```python
from build123d import *

# Parameters (mm, degrees)
F0_R     = 17.4093828925
F1_DEPTH = 25.4
F2_W     = 27.6633873582
F2_H     = 53.7356156856
F3_DEPTH = 25.4
F4_W     = 27.6633873582
F4_H     = 17.2435138375
F5_DEPTH = 12.7


with BuildPart() as f1:
    # F0 (on Top) → F1 (new body)
    with BuildSketch(Plane.XY):
        with BuildLine():
            ThreePointArc((-62.1633082628, 0), (-54.3854373577, -19.1652168316), (-35.2955013514, -27.1260682493))
            Line((-35.2955013514, -27.1260682493), (41.6988097131, -27.1260682493))
            Line((41.6988097131, -27.1260682493), (41.6988097131, 26.6095474362))
            Line((41.6988097131, 26.6095474362), (-35.6965139508, 26.6095474362))
            ThreePointArc((-35.6965139508, 26.6095474362), (-54.3456505922, 18.6914592057), (-62.1633082628, 0))
        make_face()
        with Locations((-35.2949523061, -0.2570371656)):
            Circle(F0_R, mode=Mode.SUBTRACT)
    extrude(amount=F1_DEPTH)

    # F2 (on face) → F3 (join)
    with BuildSketch(Plane(origin=(0, 0, 0), x_dir=(1, 0, 0), z_dir=(0, 0, -1))):
        with Locations((27.867116034, 0.2582604066)):
            Rectangle(F2_W, F2_H)
    extrude(amount=F3_DEPTH)

    # F4 (on face) → F5 (cut)
    with BuildSketch(Plane(origin=(0, 0, -25.4), x_dir=(1, 0, 0), z_dir=(0, 0, -1))):
        with Locations((27.867116034, 18.5043113306)):
            Rectangle(F4_W, F4_H)
    extrude(amount=-F5_DEPTH, mode=Mode.SUBTRACT)


solid = f1.part
```
For this review, take the finished solid that the model builds, in its own axes (mm). A direction names the side the tool comes from. Coordinates: 2 decimals unless noted, no trailing zeros. Write each loop counter-clockwise with the first axis right and the second up, starting at its lowest first coordinate (ties: lowest second). Pieces come first, ordered by that corner, then holes. Notation, with made-up numbers: (6.5, 2.25) -> (19.5, 2.25) arc R27 cw to (19.5, 25.25) -> close; hole circle Ø11 at (38, 15). An arc over 180 degrees is marked (long way). Put each result on its own line as item: value.
Q1. Take a section at C-C, the plane z = 4. State the section outline as (x, y) points.
From the geometry:
outline: (-62.16, 0) arc R26.87 ccw to (-35.3, -27.13) -> (41.7, -27.13) -> (41.7, 26.61) -> (-35.7, 26.61) arc R26.87 ccw to start; hole circle Ø34.82 at (-35.29, -0.26)
Q2. Clearance check with flat-ended pins moving along their axes: pin 1 Ø10 at (x, z) = (12, -13) entering from -Y; pin 2 Ø1.5 at (x, y) = (12, 11) entering from -Z; pin 3 Ø12.5 at (y, z) = (-2, -11) entering from -X; pin 4 Ø1.5 at (y, z) = (2.5, 8) entering from -X. State where each tip first meets the part, or that it passes through.
From the geometry:
pin 1: stops at y = -27.13
pin 2: stops at z = 0
pin 3: stops at x = 14.04
pin 4: stops at x = -62.09
Q3. Tool access review of faces 5 (the flat face through (28, 8, -25.4)), 6 (the flat face through (28, -9.883, -19)), 7 (the flat face through (-16, 0, 0)): name each direction out of +Z, -Z, +X, -X, +Y, -Y from which nothing blocks a thin tool from reaching the whole face with its end or side.
From the geometry:
face 5: -Z, +X, -X, +Y, -Y
face 6: -Z, +X, -X, -Y
face 7: -Z, -X, +Y, -Y
Q4. Take a section at D-D, the plane y = 15.5. State the section outline as (x, z) points.
From the geometry:
outline: (-57.06, 0) -> (-42.7, 0) -> (-42.7, 25.4) -> (-57.06, 25.4) -> close; (-27.89, 0) -> (14.04, 0) -> (14.04, -25.4) -> (41.7, -25.4) -> (41.7, 25.4) -> (-27.89, 25.4) -> close
Q5. Take a section at A-A, the plane y = -14. State the section outline as (x, z) points, then the cut area to 3 significant figures.
From the geometry:
outline: (-58.38, 0) -> (-45.98, 0) -> (-45.98, 25.4) -> (-58.38, 25.4) -> close; (-24.61, 0) -> (14.04, 0) -> (14.04, -12.7) -> (41.7, -12.7) -> (41.7, 25.4) -> (-24.61, 25.4) -> close
area: 2,350 mm2
Q6. Take a section at B-B, the plane x = -33. State the section outline as (y, z) points, then the cut area to 3 significant figures.
From the geometry:
outline: (-27.13, 0) -> (-17.51, 0) -> (-17.51, 25.4) -> (-27.13, 25.4) -> close; (17, 0) -> (26.61, 0) -> (26.61, 25.4) -> (17, 25.4) -> close
area: 488 mm2
Q7. The part is to be moulded in two halves that separate along X. For faces 1 (the flat face through (14.035, 6, -13)), 2 (the cylindrical face through (-49.11, -10.85, 12.52)), 3 (the flat face through (28, -19, -12.7)), 4 (the flat face through (41.699, 0, 0)), say which applies: +X half, -X half, draft (parallel to the pull), parting line (faces both ways), or undercut.
From the geometry:
face 1: -X half
face 2: undercut
face 3: draft
face 4: +X half
Q8. Wall thickness on L1, parallel to Z at x = 13, y = 0; L2, parallel to Z at x = 37, y = -19.5; L3, parallel to Y at x = 26.5, z = -16.5: over which ranges is each line inside the solid? List them lowest first.
From the geometry:
L1: z = 0 to 25.4
L2: z = -12.7 to 25.4
L3: y = -9.88 to 26.61
